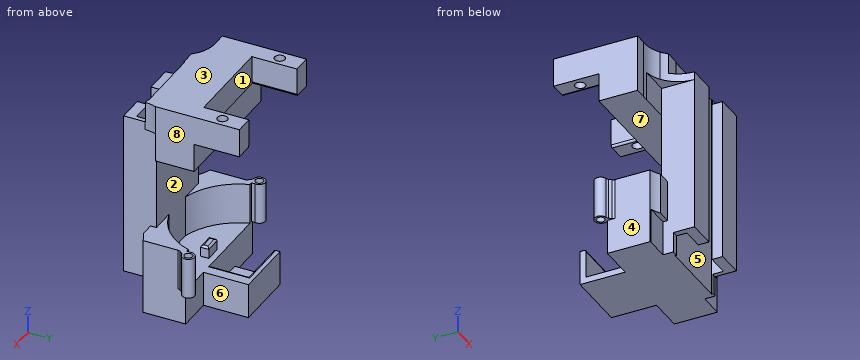
```python
from build123d import *

# Parameters (mm, degrees)
BOSS_EXTRUDE1_DEPTH = 50
SKETCH2_R           = 1.25
BOSS_EXTRUDE2_DEPTH = 7
FILLET1_R           = 8
BOSS_EXTRUDE3_DEPTH = 8.5
SKETCH7_W           = 12
SKETCH7_H           = 9.5
CUT_EXTRUDE1_DEPTH  = 7
BOSS_EXTRUDE4_DEPTH = 10
SKETCH9_W           = 3.98
SKETCH9_H           = 1.98
BOSS_EXTRUDE5_DEPTH = 2.8
SKETCH11_W          = 32
SKETCH11_H          = 9.453112349
BOSS_EXTRUDE6_DEPTH = 7
SKETCH16_R          = 1
BOSS_EXTRUDE7_DEPTH = 10
FILLET2_R           = 1
FILLET4_R           = 0.5
FILLET5_R           = 0.5
FILLET6_R           = 0.5
SKETCH17_R          = 8
CUT_EXTRUDE2_DEPTH  = 61.270972563
SKETCH18_W          = 26.905399266
SKETCH18_H          = 5.924124609
CUT_EXTRUDE3_DEPTH  = 5
SKETCH19_W          = 27.645914842
SKETCH19_H          = 7.775413549
CUT_EXTRUDE4_DEPTH  = 5


with BuildPart() as part:
    # Sketch1 → Boss-Extrude1 (new body)
    with BuildSketch(Plane.XY):
        Polygon((-6.349640288, 0), (-0.949640288, 0), (-0.949640288, -2.6), (-7.849640288, -2.6), (-7.849640288, 5.4), (12.150359712, 5.4), (12.150359712, -2.6), (5.650359712, -2.6), (5.650359712, 0), (11.050359712, 0), (11.050359712, 2.9), (-6.349640288, 2.9), align=None)
    extrude(amount=BOSS_EXTRUDE1_DEPTH)

    # Sketch2 → Boss-Extrude2 (add)
    with BuildSketch(Plane.XY.offset(50)):
        Polygon((-19.349640288, 25.9), (-19.349640288, 5.4), (12.650359712, 5.4), (12.650359712, 25.9), (8.150359712, 25.9), (8.150359712, 14.9), (-14.849640288, 14.9), (-14.849640288, 25.9), align=None)
        with Locations((10.350359712, 20.6)):
            Circle(SKETCH2_R, mode=Mode.SUBTRACT)
        with Locations((-17.049640288, 20.6)):
            Circle(SKETCH2_R, mode=Mode.SUBTRACT)
    extrude(amount=-BOSS_EXTRUDE2_DEPTH)

    # Fillet1
    # the kernel refuses this fillet: 8 mm, written as the material it adds along each edge
    with BuildSketch(Plane(origin=(-7.849640288, 5.4, 43), x_dir=(0, -1, 0), z_dir=(0, 0, 1))) as fillet1_piece_1:
        with BuildLine():
            CenterArc((FILLET1_R, -FILLET1_R), FILLET1_R, 90, 90)
            Line((0, -FILLET1_R), (0, 0))
            Line((0, 0), (FILLET1_R, 0))
        make_face()
    extrude(amount=7)
    with BuildSketch(Plane(origin=(12.150359712, 5.4, 43), x_dir=(0, -1, 0), z_dir=(0, 0, 1))) as fillet1_piece_2:
        with BuildLine():
            CenterArc((2.783882181, 8), FILLET1_R, 249.635865194, 20.364134806)
            Line((0, 0.5), (0, 0))
            Line((0, 0), (2.783882181, 0))
        make_face()
    extrude(amount=7)

    # Sketch4 → Boss-Extrude3 (add)
    with BuildSketch(Plane(origin=(0, 0, 0), x_dir=(-1, 0, 0), z_dir=(0, 0, -1))):
        Polygon((-18.150359712, 15.6), (-18.150359712, 5.1), (13.849640288, 5.1), (13.849640288, 15.6), (5.349640288, 15.6), (5.349640288, 26.6), (-9.650359712, 26.6), (-9.650359712, 15.6), align=None)
    extrude(amount=-BOSS_EXTRUDE3_DEPTH)

    # Sketch7 → Cut-Extrude1 (cut)
    with BuildSketch(Plane.XY.offset(8.5)):
        with Locations((0.650359712, 20.35)):
            Rectangle(SKETCH7_W, SKETCH7_H)
    extrude(amount=-CUT_EXTRUDE1_DEPTH, mode=Mode.SUBTRACT)

    # Sketch8 → Boss-Extrude4 (add)
    with BuildSketch(Plane.XY.offset(8.5)):
        with BuildLine():
            Line((-13.849640288, 15.6), (-12.587686291, 15.6))
            ThreePointArc((-12.587686291, 15.6), (2.150359712, 4.9), (16.888405716, 15.6))
            Line((16.888405716, 15.6), (18.150359712, 15.6))
            Line((18.150359712, 15.6), (18.150359712, 3.937972429))
            Line((18.150359712, 3.937972429), (-13.849640288, 3.937972429))
            Line((-13.849640288, 3.937972429), (-13.849640288, 15.6))
        make_face()
    extrude(amount=BOSS_EXTRUDE4_DEPTH)

    # Sketch9 → Boss-Extrude5 (add)
    with BuildSketch(Plane.XY.offset(8.5)):
        with Locations((2.150359712, 13.1)):
            Rectangle(SKETCH9_W, SKETCH9_H)
    extrude(amount=BOSS_EXTRUDE5_DEPTH)

    # Sketch11 → Boss-Extrude6 (add)
    with BuildSketch(Plane(origin=(0, 0, 43), x_dir=(-1, 0, 0), z_dir=(0, 0, -1))):
        with Locations((3.349640288, 10.126556175)):
            Rectangle(SKETCH11_W, SKETCH11_H)
    extrude(amount=BOSS_EXTRUDE6_DEPTH)

    # Sketch16 → Boss-Extrude7 (add)
    # profile 1 of 2: a face of its own
    with BuildSketch(Plane.XY.offset(18.5)):
        with BuildLine():
            Line((-13.346805139, 15.601949196), (-13.846805139, 15.601949196))
            Line((-13.846805139, 15.601949196), (-13.849640288, 14.1))
            Line((-13.849640288, 14.1), (-14.815015575, 15.247623037))
            ThreePointArc((-14.815015575, 15.247623037), (-15.7608574, 17.911832315), (-13.346805139, 16.44044538))
            Line((-13.346805139, 16.44044538), (-13.346805139, 15.601949196))
        make_face()
        with Locations((-14.815015575, 16.747623037)):
            Circle(SKETCH16_R, mode=Mode.SUBTRACT)
    # profile 2 of 2: a face of its own
    with BuildSketch(Plane.XY.offset(18.5)):
        with BuildLine():
            Line((17.652000257, 15.6), (18.150359712, 15.6))
            Line((18.150359712, 15.6), (18.150359712, 14.1))
            Line((18.150359712, 14.1), (19.116258964, 15.247623037))
            ThreePointArc((19.116258964, 15.247623037), (20.054810716, 17.91771731), (17.652000257, 16.422128892))
            Line((17.652000257, 16.422128892), (17.652000257, 15.6))
        make_face()
        with Locations((19.116258964, 16.747623037)):
            Circle(SKETCH16_R, mode=Mode.SUBTRACT)
    extrude(amount=-BOSS_EXTRUDE7_DEPTH)

    # Fillet2
    fillet2_edges = [part.edges().sort_by_distance(p)[0] for p in [
        (-13.849640288, 14.1, 13.5),
        (-14.815015575, 15.247623037, 13.5),
        (19.116258964, 15.247623037, 13.5),
        (18.150359712, 14.1, 13.5),
    ]]
    fillet(fillet2_edges, radius=FILLET2_R)

    # Fillet4
    fillet4_edges = [part.edges().sort_by_distance(p)[0] for p in [
        (0.160359712, 13.1, 11.3),
        (2.150359712, 12.11, 11.3),
        (4.140359712, 13.1, 11.3),
        (2.150359712, 14.09, 11.3),
    ]]
    fillet(fillet4_edges, radius=FILLET4_R)

    # Fillet5
    fillet5_edges = [part.edges().sort_by_distance(p)[0] for p in [
        (6.650359712, 20.35, 8.5),
        (0.650359712, 25.1, 8.5),
    ]]
    fillet(fillet5_edges, radius=FILLET5_R)

    # Fillet6
    fillet6_edges = [part.edges().sort_by_distance(p)[0] for p in [
        (-14.849640288, 20.4, 43),
        (8.150359712, 20.4, 43),
    ]]
    fillet(fillet6_edges, radius=FILLET6_R)

    # Sketch17 → Cut-Extrude2 (cut, through all)
    with BuildSketch(Plane.XY.offset(50)):
        with Locations((-15.895053234, -2.569483857)):
            Circle(SKETCH17_R)
        with Locations((20.210973801, -2.569483857)):
            Circle(SKETCH17_R)
    extrude(amount=-CUT_EXTRUDE2_DEPTH, mode=Mode.SUBTRACT)

    # Sketch18 → Cut-Extrude3 (cut)
    with BuildSketch(Plane.XY.offset(50)):
        with Locations((1.903783169, -0.265657621)):
            Rectangle(SKETCH18_W, SKETCH18_H)
    extrude(amount=-CUT_EXTRUDE3_DEPTH, mode=Mode.SUBTRACT)

    # Sketch19 → Cut-Extrude4 (cut)
    with BuildSketch(Plane(origin=(0, 0, 0), x_dir=(-1, 0, 0), z_dir=(0, 0, -1))):
        with Locations((-1.944922923, -1.314721353)):
            Rectangle(SKETCH19_W, SKETCH19_H)
    extrude(amount=-CUT_EXTRUDE4_DEPTH, mode=Mode.SUBTRACT)


solid = part.part
```
Geometry check sheet. Reference: the model listing, model coordinates, mm. Face numbers are marked on the shaded views. A direction names the side the tool comes from. Give positions to 0.01 mm unless a question says otherwise; leave off trailing zeros. Loops run counter-clockwise (first coordinate to the right, second up) from the corner with the lowest first, then second, coordinate; pieces in that order, holes last. Notation, with made-up numbers: (60.25, 27) - (94.25, 27) arc R23 cw to (94.25, 37) - close; hole circle Ø6 at (33, 28). An arc over 180 degrees is marked (long way). Use CSV: the item, a comma, the result in double quotes. Start each with the question number.
Q1. Section check B-B, the plane x = 5. Record the cut outline in (y, z), and give its area (3 significant figures).
Q2. Scan lines: probe 1 along Y at (x, z) = (7, 27); probe 2 along Z at (x, y) = (-10, 12); probe 3 along X at (y, z) = (0.5, 36.5). Record each from-to range of solid material in increasing order. Write a range as from..to.
Q3. Go/stop test with flat-tipped pins: pin 1 Ø2.5 at (x, y) = (-4, -1) entering from -Z; pin 2 Ø7 at (y, z) = (19, 43) entering from +X; pin 3 Ø4.5 at (x, z) = (8.5, 21) entering from +Y; pin 4 Ø1.8 at (x, y) = (19.12, 16.75) entering from +Z. Record where each tip stops, or that it passes through.
Q4. Section check D-D, the plane z = 14.5. Count the separate pieces of the cut face and the enclosed holes in it, and give its area (3 significant figures).
Q5. Section check C-C, the plane z = 29. Record the cut outline in (x, y).
Q6. Release check for a two-part mould opening along Z. For the marked faces 1, 2 and 3 record: +Z half, -Z half, draft (parallel to the pull), parting line (faces both ways), or undercut.
Q7. Access from +Z, -Z, +X, -X, +Y, -Y to the whole of each face (thin tool, end or side, straight path). Record for the marked faces 4, 5, 6, 7 and 8.
Q8. Section check A-A, the plane y = 20.6. Record the cut outline in (x, z), and give its area (3 significant figures).
Findings below:
1,outline,"(2.9, 0) - (26.6, 0) - (26.6, 8.5) - (25.6, 8.5) arc R0.5 ccw to (25.1, 8) - (25.1, 1.5) - (15.6, 1.5) - (15.6, 8.5) - (5.4, 8.5) - (5.4, 36) - (14.85, 36) - (14.85, 43) - (14.9, 43) - (14.9, 50) - (2.9, 50) - close"
1,area,"371 mm^2"
2,probe 1,"y = -2.6..0, 2.9..5.4"
2,probe 2,"z = 0..8.5, 36..50"
2,probe 3,"x = -7.85..-6.35, 11.05..12.15"
3,pin 1,"stops at z = 5"
3,pin 2,"stops at x = 12.65"
3,pin 3,"stops at y = 5.4"
3,pin 4,"passes through"
4,separate pieces,"1"
4,enclosed holes,"2"
4,area,"214 mm^2"
5,outline,"(-7.85, -2.6) - (-0.95, -2.6) - (-0.95, 0) - (-6.35, 0) - (-6.35, 2.9) - (11.05, 2.9) - (11.05, 0) - (5.65, 0) - (5.65, -2.6) - (12.15, -2.6) - (12.15, 5.4) - (-7.85, 5.4) - close"
6,face 1,"draft"
6,face 2,"undercut"
6,face 3,"+Z half"
7,face 4,"-Z, -X, -Y"
7,face 5,"+Z, -Z"
7,face 6,"-Z, +X, +Y"
7,face 7,"+X, -X, +Y"
7,face 8,"+Z, +X, +Y, -Y"
8,outline,"(-19.35, 43) - (-18.3, 43) - (-18.3, 50) - (-19.35, 50) - close; (-15.8, 43) - (-15.35, 43) arc R0.5 ccw to (-14.85, 43.5) - (-14.85, 50) - (-15.8, 50) - close; (-5.35, 0) - (9.65, 0) - (9.65, 8.5) - (7.15, 8.5) arc R0.5 ccw to (6.65, 8) - (6.65, 1.5) - (-5.35, 1.5) - close; (8.15, 43.5) arc R0.5 ccw to (8.65, 43) - (9.1, 43) - (9.1, 50) - (8.15, 50) - close; (11.6, 43) - (12.65, 43) - (12.65, 50) - (11.6, 50) - close"
8,area,"71.3 mm^2"
